Build history of the part. All positions in model axes, mm. A direction names the side the tool comes from. Round coordinates to 2 decimals unless told otherwise and drop trailing zeros. Write each loop counter-clockwise with the first axis right and the second up, starting at its lowest first coordinate (ties: lowest second). Pieces come first, ordered by that corner, then holes. Notation, with made-up numbers: (19, 42) -> (69, 42) arc R24 cw to (69, 53) -> close; hole circle Ø8 at (-39, -10.5). An arc over 180 degrees is marked (long way). Answer in a Markdown table with one row per item. Add a question column.
from build123d import *

# Parameters (mm, degrees)
F0_R     = 10
F1_DEPTH = 30
F2_DEPTH = 60


with BuildPart() as f1:
    # F0 (on Front) → F1 (new body)
    with BuildSketch(Plane.XZ):
        with BuildLine():
            ThreePointArc((19.364917, -5), (19.840594, -2.520086), (20, 0))
            ThreePointArc((20, 0), (19.840594, 2.520086), (19.364917, 5))
            ThreePointArc((19.364917, 5), (-20, 0), (19.364917, -5))
        make_face()
        Circle(F0_R, mode=Mode.SUBTRACT)
    extrude(amount=F1_DEPTH)

    # F0 (on Front) → F2 (join)
    with BuildSketch(Plane.XZ):
        with BuildLine():
            ThreePointArc((19.364917, 5), (19.840594, 2.520086), (20, 0))
            Line((20, 0), (80, 0))
            Line((80, 0), (80, 5))
            Line((80, 5), (19.364917, 5))
        make_face()
        with BuildLine():
            Line((80, 0), (20, 0))
            ThreePointArc((20, 0), (19.840594, -2.520086), (19.364917, -5))
            Line((19.364917, -5), (80, -5))
            Line((80, -5), (80, 0))
        make_face()
    extrude(amount=F2_DEPTH)


solid = f1.part
(1) Saw through at B-B (z = 7). List the corners of the cut face in (x, y) (3 decimals), plus the area to 3 significant figures.
(2) Which spindle directions (+Z, -Z, +X, -X, +Y, -Y) get a long thin tool onto all of the face, cutting with end or side? Do faces 1 (the face through (49, -60, 0)), 2 (the face through (49, -30, -5)), 3 (the face through (50, -30, 5)). Say none if no direction does.
(3) Saw through at A-A (x = 0). List the corners of the cut face in (y, z), plus the area to 3 significant figures.
(4) Saw through at C-C (y = -5). List the corners of the cut face in (x, z), plus the area to 3 significant figures.
(5) Drop flat-ended pins along their axis: P1, Ø2, axis at y = -9, z = -13.5, coming from the +X side; P2, Ø16, axis at x = 0, z = 0, coming from the -Y side; P3, Ø12, axis at x = 54.5, y = -32, coming from the -Z side; P4, Ø8, axis at y = -29.5, z = -14.5, coming from the -X side. Give the stop position or say it passes through.
(6) Saw through at D-D (y = -37). List the corners of the cut face in (x, z).
(7) Probe line 1 along Z through (x, y) = (0, -11.5); line 2 along Y through (x, z) = (2, -13.5); line 3 along Z through (x, y) = (21.5, -35.5). List the from-to ranges inside material, lowest first.
(8) Mould opens along Z. For faces 4 (the face through (-2.17, -14.79, -9.76)), 5 (the face through (80, -30, 0)), 6 (the face through (-19.984, -14.79, 0.809)) say: pulls with the +Z half, pulls with the -Z half, needs draft (parallel to the pull), parting line crosses it, or undercut.
Answer sheet:
| question | item | result |
|---|---|---|
| 1 | outline | (-18.735, -30) -> (-7.141, -30) -> (-7.141, 0) -> (-18.735, 0) -> close; (7.141, -30) -> (18.735, -30) -> (18.735, 0) -> (7.141, 0) -> close |
| 1 | area | 696 mm² |
| 2 | face 1 | +Z, -Z, +X, -X, -Y |
| 2 | face 2 | -Z, +X, +Y, -Y |
| 2 | face 3 | +Z, +X, +Y, -Y |
| 3 | outline | (-30, -20) -> (0, -20) -> (0, -10) -> (-30, -10) -> close; (-30, 10) -> (0, 10) -> (0, 20) -> (-30, 20) -> close |
| 3 | area | 600 mm² |
| 4 | outline | (19.36, -5) -> (80, -5) -> (80, 5) -> (19.36, 5) arc R20 ccw (long way) to start; hole circle Ø20 at (0, 0) |
| 4 | area | 1,540 mm² |
| 5 | P1 | stops at x = 15.61 |
| 5 | P2 | passes through |
| 5 | P3 | stops at z = -5 |
| 5 | P4 | stops at x = -17.02 |
| 6 | outline | (19.36, -5) -> (80, -5) -> (80, 5) -> (19.36, 5) arc R20 cw to start |
| 7 | line 1 | z = -20 to -10, 10 to 20 |
| 7 | line 2 | y = -30 to 0 |
| 7 | line 3 | z = -5 to 5 |
| 8 | face 4 | undercut |
| 8 | face 5 | needs draft |
| 8 | face 6 | parting line crosses it |
